from build123d import *

# Parameters (mm, degrees)
F0_R     = 25.4
F0_R_2   = 23.495
F1_DEPTH = 50.8
F3_D     = 45.72


# Not quite as in the source:
# - a fillet or chamfer that OpenCascade refuses, or shapes differently, is made with other operations: its cross-section is extruded or revolved along the edge and cut away or added


with BuildPart() as f1:
    # F0 (on Front) → F1 (new body, symmetric)
    with BuildSketch(Plane.XZ):
        Circle(F0_R)
        Circle(F0_R_2, mode=Mode.SUBTRACT)
        Circle(F0_R_2)
    extrude(amount=F1_DEPTH, both=True)

    # F3 (through all)
    with Locations(Plane.XZ.offset(50.8)):
        with Locations((0, 0)):
            Hole(F3_D / 2)

    # F4: chamfer of 5.08 on 3 edges, made by hand

    # F4_s1 → F4_t2 (revolve, cut)
    with BuildSketch(Plane.XY):
        Polygon((25.4, 45.72), (20.32, 50.8), (25.4, 50.8), align=None)
    revolve(axis=Axis((0, 50.8, 0), (0, -1, 0)), mode=Mode.SUBTRACT)

    # F4_s3 → F4_t4 (revolve, cut)
    with BuildSketch(Plane.XY):
        Polygon((25.4, -45.72), (20.32, -50.8), (25.4, -50.8), align=None)
    revolve(axis=Axis((0, -50.8, 0), (0, -1, 0)), mode=Mode.SUBTRACT)


solid = f1.part
Read the model definition and answer for the solid it produces. Units are mm, in the model's axes. Coordinates: 2 decimals unless noted, no trailing zeros. Loops run counter-clockwise (first coordinate to the right, second up) from the corner with the lowest first, then second, coordinate; pieces in that order, holes last. Notation, with made-up numbers: (42, -15) -> (96, -15) arc R11 cw to (96, -11) -> close; hole circle Ø11 at (72.25, -22). An arc over 180 degrees is marked (long way). Answer in a Markdown table with one row per item.
Item 1: Each of these flat-tipped pins is pushed along its axis until it touches: P1, Ø1, axis at x = -11, y = -31, coming from the -Z side; P2, Ø4, axis at x = 16.5, y = -2.5, coming from the +Z side; P3, Ø3, axis at x = -0.5, y = -11, coming from the -Z side. Where does it stop, or does it pass through?
Returned:
| item | result |
|---|---|
| P1 | stops at z = -23.13 |
| P2 | stops at z = 20.85 |
| P3 | stops at z = -25.4 |
Item 2: For a pull along X with two mould halves and no side action, classify faces 1 (the conical face through (-23, 48.1, 1)), 2 (the cylindrical face through (-21.804, 0.676, 6.867)) as released by +X, released by -X, zero draft, split by the parting line, or undercut.
Returned:
| item | result |
|---|---|
| face 1 | split by the parting line |
| face 2 | undercut |
Item 3: Straight lines are drawn through the part: line 1 along Z through (x, y) = (0, -6); line 2 along Z through (x, y) = (-17.5, -40); line 3 along X through (y, z) = (-14, 16). For each, find the intervals that lie inside material, in ascending order. Write a range as [from, to].
Returned:
| item | result |
|---|---|
| line 1 | z = [-25.4, -22.86], [22.86, 25.4] |
| line 2 | z = [-18.41, -14.71], [14.71, 18.41] |
| line 3 | x = [-19.73, -16.33], [16.33, 19.73] |
Item 4: A cutting plane is placed at B-B on x = 0. Determine the outline of the cut face in (y, z).
Returned:
| item | result |
|---|---|
| outline | (-48.26, -22.86) -> (-45.72, -25.4) -> (45.72, -25.4) -> (48.26, -22.86) -> close; (-48.26, 22.86) -> (48.26, 22.86) -> (45.72, 25.4) -> (-45.72, 25.4) -> close |
Item 5: A cutting plane is placed at C-C on y = 15. Determine the outline of the cut face in (x, z), plus the area to 3 significant figures.
Returned:
| item | result |
|---|---|
| outline | circle Ø50.8 at (0, 0); hole circle Ø45.72 at (0, 0) |
| area | 385 mm^2 |
Item 6: A cutting plane is placed at A-A on z = 0. Determine the outline of the cut face in (x, y).
Returned:
| item | result |
|---|---|
| outline | (-25.4, -45.72) -> (-22.86, -48.26) -> (-22.86, 48.26) -> (-25.4, 45.72) -> close; (22.86, -48.26) -> (25.4, -45.72) -> (25.4, 45.72) -> (22.86, 48.26) -> close |
